CAD build for the part. Positions are in the model's coordinates, mm. A direction names the side the tool comes from. Coordinates: 2 decimals unless noted, no trailing zeros. Loops run counter-clockwise (first coordinate to the right, second up) from the corner with the lowest first, then second, coordinate; pieces in that order, holes last.
1) Wall check: line 1 along X through (y, z) = (-9.3, -10.7); line 2 along Z through (x, y) = (-7.75, 3.5) (3 decimals); line 3 along Y through (x, z) = (-5.25, -18.25) (3 decimals). Give the ranges that are in metal, low to high.
2) Saw through at B-B, the plane z = -10.7. Write the cut outline in (x, y) (3 decimals), and give its area (4 significant figures).
3) Which spindle directions (+Z, -Z, +X, -X, +Y, -Y) get a long thin tool onto all of the face, cutting with end or side? Do faces 1 (the flat face through (6.5, -9.5, -24)), 2 (the flat face through (0, -1, 0)). Say none if no direction does.
4) Two-plate mould, pull along Y, no slides. Class faces 3 (the cylindrical face through (-10.5, 0.07, 0.32)), 4 (the flat face through (-12.5, -3.9, 0.2)), 5 (the cylindrical face through (7.8, -0.9, 0.3)), 6 (the flat face through (3, -9.765, -13)): +Y half, -Y half, draft (parallel to the pull), parting line (faces both ways), or undercut.
5) Saw through at D-D, the plane z = -18.5. Write the cut outline in (x, y) (3 decimals), and give its area (4 significant figures).
6) Pin check, flat tips, straight feed: pin 1 Ø5 at (x, z) = (-9.5, -14) entering from +Y; pin 2 Ø2.5 at (x, y) = (9, 0) entering from -Z; pin 3 Ø0.7 at (y, z) = (-9.5, -9.5) entering from -X. Stop position of each tip, or through.
7) Saw through at A-A, the plane y = 0. Write the cut outline in (x, z) (3 decimals), and give its area (3 significant figures).
8) Saw through at C-C, the plane x = -9. Write the cut outline in (y, z) (3 decimals), and give its area (3 significant figures).
```python
from build123d import *

# Parameters (mm, degrees)
BASE_FLANGE1_DEPTH        = 12.5
SKETCH7_R                 = 4
CUT_EXTRUDE1_DEPTH        = 10
SKETCH8_R                 = 1.5
CUT_EXTRUDE2_DEPTH        = 0.635
BREAK_CORNER1_START       = 11.66726189
BREAK_CORNER1_OUTLINE_W   = 6
BREAK_CORNER1_OUTLINE_H   = 3
BREAK_CORNER1_DEPTH       = 1.414213562
BREAK_CORNER1_START_2     = 21.566756826
BREAK_CORNER1_2_OUTLINE_W = 14
BREAK_CORNER1_2_OUTLINE_H = 3
BREAK_CORNER1_2_DEPTH     = 1.414213563
BREAK_CORNER1_START_3     = -22.980970389
BREAK_CORNER1_3_OUTLINE_W = 14
BREAK_CORNER1_3_OUTLINE_H = 3
BREAK_CORNER1_3_DEPTH     = 1.414213563
BREAK_CORNER1_START_4     = -13.081475452
BREAK_CORNER1_4_OUTLINE_W = 6
BREAK_CORNER1_4_OUTLINE_H = 3
BREAK_CORNER1_4_DEPTH     = 1.414213562


# Read off the part's stored shape, not the designer's step: Break-Corner1
# Sheet-metal steps are written as plain solids
with BuildPart() as part:
    # Sketch2 → Base-Flange1 (new, symmetric)
    with BuildSketch(Plane(origin=(0, 0, 0), x_dir=(0, 0, -1), z_dir=(1, 0, 0))):
        with BuildLine():
            Line((0, 6), (0, -8.749))
            ThreePointArc((0, -8.749), (0.111592316, -9.018407684), (0.381, -9.13))
            Line((0.381, -9.13), (25, -9.13))
            Line((25, -9.13), (25, -9.765))
            Line((25, -9.765), (0.381, -9.765))
            ThreePointArc((0.381, -9.765), (-0.33742049, -9.46742049), (-0.635, -8.749))
            Line((-0.635, -8.749), (-0.635, 6))
            Line((-0.635, 6), (0, 6))
        make_face()
    extrude(amount=BASE_FLANGE1_DEPTH, both=True)

    # Sketch7 → Cut-Extrude1 (cut)
    with BuildSketch(Plane.XZ.offset(9.765)):
        with Locations(Location((-1.007441433, -10.7, 0), (0, 0, 270))):
            Circle(SKETCH7_R)
        Polygon((7.5, -25), (7.5, -5), (12.5, -2.113248654), (12.5, -25), align=None)
        Polygon((-7.5, -25), (-7.5, -5), (-12.5, -2.113248654), (-12.5, -25), align=None)
    extrude(amount=-CUT_EXTRUDE1_DEPTH, mode=Mode.SUBTRACT)

    # Sketch8 → Cut-Extrude2 (cut)
    with BuildSketch(Plane.XY.offset(0.635)):
        with Locations((9, 0)):
            Circle(SKETCH8_R)
        with Locations((-9, 0)):
            Circle(SKETCH8_R)
    extrude(amount=-CUT_EXTRUDE2_DEPTH, mode=Mode.SUBTRACT)

    # Break-Corner1 outline → Break-Corner1 (cut)
    with BuildSketch(Plane(origin=(0, 0, 0), x_dir=(0.7071067811865474, -0.7071067811865477, 0), z_dir=(0.7071067811865476, 0.7071067811865476, 0)).offset(BREAK_CORNER1_START)):
        with Locations((5, -0.5)):
            Rectangle(BREAK_CORNER1_OUTLINE_W, BREAK_CORNER1_OUTLINE_H)
    extrude(amount=BREAK_CORNER1_DEPTH, mode=Mode.SUBTRACT)

    # Break-Corner1 2 outline → Break-Corner1 2 (cut)
    with BuildSketch(Plane(origin=(0, 0, 0), x_dir=(0.707106781186548, 0, 0.707106781186547), z_dir=(0.707106781186547, 0, -0.707106781186548)).offset(BREAK_CORNER1_START_2)):
        with Locations((-16, 9.5)):
            Rectangle(BREAK_CORNER1_2_OUTLINE_W, BREAK_CORNER1_2_OUTLINE_H)
    extrude(amount=BREAK_CORNER1_2_DEPTH, mode=Mode.SUBTRACT)

    # Break-Corner1 3 outline → Break-Corner1 3 (cut)
    with BuildSketch(Plane(origin=(0, 0, 0), x_dir=(0.7071067811865474, 0, -0.7071067811865477), z_dir=(0.7071067811865476, 0, 0.7071067811865476)).offset(BREAK_CORNER1_START_3)):
        with Locations((16, -9.5)):
            Rectangle(BREAK_CORNER1_3_OUTLINE_W, BREAK_CORNER1_3_OUTLINE_H)
    extrude(amount=BREAK_CORNER1_3_DEPTH, mode=Mode.SUBTRACT)

    # Break-Corner1 4 outline → Break-Corner1 4 (cut)
    with BuildSketch(Plane(origin=(0, 0, 0), x_dir=(0.707106781186548, 0.707106781186547, 0), z_dir=(0.707106781186547, -0.707106781186548, 0)).offset(BREAK_CORNER1_START_4)):
        with Locations((-5, 0.5)):
            Rectangle(BREAK_CORNER1_4_OUTLINE_W, BREAK_CORNER1_4_OUTLINE_H)
    extrude(amount=BREAK_CORNER1_4_DEPTH, mode=Mode.SUBTRACT)


solid = part.part
```
Data:
1. line 1: x = -7.5 to -5.01, 2.99 to 7.5
1. line 2: z = 0 to 0.635
1. line 3: y = -9.765 to -9.13
2. outline: (-7.5, -9.765) - (-5.007, -9.765) - (-5.007, -9.13) - (-7.5, -9.13) - close; (2.993, -9.765) - (7.5, -9.765) - (7.5, -9.13) - (2.993, -9.13) - close
2. area: 4.445 mm2
3. face 1: -Z, +X, +Y, -Y
3. face 2: -Z, +X, -X, +Y
4. face 3: undercut
4. face 4: draft
4. face 5: undercut
4. face 6: -Y half
5. outline: (-7.5, -9.765) - (7.5, -9.765) - (7.5, -9.13) - (-7.5, -9.13) - close
5. area: 9.525 mm2
6. pin 1: stops at y = -9.13
6. pin 2: passes through
6. pin 3: stops at x = -7.5
7. outline: (-12.5, 0) - (-10.5, 0) - (-10.5, 0.635) - (-12.5, 0.635) - close; (-7.5, 0) - (7.5, 0) - (7.5, 0.635) - (-7.5, 0.635) - close; (10.5, 0) - (12.5, 0) - (12.5, 0.635) - (10.5, 0.635) - close
7. area: 12.1 mm2
8. outline: (-9.765, -4.134) - (-9.13, -4.134) - (-9.13, -0.381) arc R0.381 cw to (-8.749, 0) - (-1.5, 0) - (-1.5, 0.635) - (-8.749, 0.635) arc R1.016 ccw to (-9.765, -0.381) - close; (1.5, 0) - (6, 0) - (6, 0.635) - (1.5, 0.635) - close
8. area: 10.5 mm2
